CAD build for the part. Positions are in the model's coordinates, mm. A direction names the side the tool comes from. Coordinates: 2 decimals unless noted, no trailing zeros. Order: outer loops, then holes, each group sorted by start corner. A loop starts at its lowest first (then second) coordinate and runs counter-clockwise, first axis right, second up. Notation, with made-up numbers: (2, 20.5) - (39, 20.5) arc R28 cw to (39, 57.5) - close; hole circle Ø5 at (16.25, -10.5). An arc over 180 degrees is marked (long way). Use one line per item in the form item = value.
```python
from build123d import *

# Parameters (mm, degrees)
EXTRUDE_1_DEPTH     = 3
EXTRUDE_2_DEPTH     = 4
CUT_EXTRUDE_1_DEPTH = 4


with BuildPart() as part:
    # 草圖1 → 填料-伸長1 (new body)
    with BuildSketch(Plane.XY):
        Polygon((0, 0), (4, 0), (3, 1), (2, 1), (2, 4), (0, 4), align=None)
    extrude_1 = extrude(amount=EXTRUDE_1_DEPTH)

    # 草圖2 → 填料-伸長2 (add)
    with BuildSketch(Plane.XY):
        with BuildLine():
            ThreePointArc((0, 2), (1.414213562, 2.585786438), (2, 4))
            Line((2, 4), (1, 4))
            ThreePointArc((1, 4), (0.707106781, 3.292893219), (0, 3))
            Line((0, 3), (0, 2))
        make_face()
    extrude_2 = extrude(amount=EXTRUDE_2_DEPTH)

    # 草圖2<3> → 除料-伸長1 (cut)
    with BuildSketch(Plane.XY):
        with BuildLine():
            ThreePointArc((0, 3), (0.707106781, 3.292893219), (1, 4))
            Line((1, 4), (0, 4))
            Line((0, 4), (0, 3))
        make_face()
    cut_extrude_1 = extrude(amount=CUT_EXTRUDE_1_DEPTH, mode=Mode.SUBTRACT)

    # 鏡射1: 填料-伸長1, 填料-伸長2, 除料-伸長1 across plane
    add(extrude_1.mirror(Plane(origin=(0, 0, 0), x_dir=(0, 0, 1), z_dir=(1, 0, 0))))
    add(extrude_2.mirror(Plane(origin=(0, 0, 0), x_dir=(0, 0, 1), z_dir=(1, 0, 0))))
    add(cut_extrude_1.mirror(Plane(origin=(0, 0, 0), x_dir=(0, 0, 1), z_dir=(1, 0, 0))), mode=Mode.SUBTRACT)


solid = part.part
```
Item 1: Drop flat-ended pins along their axis: pin 1 (1.1 mm diameter, centred on x = -2.5, z = 1.5, fed in from +Y); pin 2 (0.8 mm diameter, centred on x = 2.5, z = 2, fed in from +Y); pin 3 (0.9 mm diameter, centred on y = 2, z = 1, fed in from +X). Give the stop position or say it passes through.
Derived:
pin_1 = 4
pin_2 = 1
pin_3 = 2
Item 2: Cut at C-C, the plane x = -3.5. Write the cut outline in (y, z), plus the area to 3 significant figures.
Derived:
outline = (0, 0) - (0.5, 0) - (0.5, 3) - (0, 3) - close
area = 1.50 mm²
Item 3: Cut at B-B, the plane z = 3.2. Write the cut outline in (x, y).
Derived:
outline = (-2, 4) arc R2 ccw to (2, 4) - (1, 4) arc R1 cw to (-1, 4) - close
Item 4: Cut at A-A, the plane y = 3.45. Write the cut outline in (x, z).
Derived:
outline = (-2, 0) - (-0.84, 0) - (-0.84, 4) - (-1.92, 4) - (-1.92, 3) - (-2, 3) - close; (0.84, 0) - (2, 0) - (2, 3) - (1.92, 3) - (1.92, 4) - (0.84, 4) - close
Item 5: Drill centre lines: line 1 (X direction, y = 1.05, z = 2.8); line 2 (Y direction, x = 0, z = 0.8); line 3 (X direction, y = 3.25, z = 3.45). Where is each one in solid material? Low to high. Write a range as [from, to].
Derived:
line_1 = [-2, 2]
line_2 = [0, 3]
line_3 = [-1.85, -0.66], [0.66, 1.85]
Item 6: 3-axis set-ups, long thin cutter, end or side, ignore diameter. For faces 1 (the face through (2, 2, 1)), 2 (the face through (-2.5, 1, 1.5)), 3 (the face through (0, 2, 0)): which of +Z, -Z, +X, -X, +Y, -Y reach the whole face in a straight line?
Derived:
face_1 = +Z, -Z, +X, +Y
face_2 = +Z, -Z, -X, +Y
face_3 = -Z, +X, -X, +Y, -Y
Item 7: Cut at D-D, the plane y = 2.75. Write the cut outline in (x, z).
Derived:
outline = (-2, 0) - (2, 0) - (2, 3) - (1.56, 3) - (1.56, 4) - (-1.56, 4) - (-1.56, 3) - (-2, 3) - close
